Work out the finished part from the listing and answer in its coordinate system (mm). Face numbers are marked on the shaded views. A direction names the side the tool comes from. Coordinates: 2 decimals unless noted, no trailing zeros. Order: outer loops, then holes, each group sorted by start corner. A loop starts at its lowest first (then second) coordinate and runs counter-clockwise, first axis right, second up. Notation, with made-up numbers: (66, -21.75) - (93, -21.75) arc R22 ccw to (93, -2.75) - close; hole circle Ø7 at (75, 43.5). An arc over 180 degrees is marked (long way). Use CSV: the item, a comma, the result in double quotes. Start each with the question number.
from build123d import *

# Parameters (mm, degrees)
SKETCH1_R                 = 1.45
BOSS_EXTRUDE1_DEPTH       = 3
SKETCH4_W                 = 3.5
SKETCH4_H                 = 12
BOSS_EXTRUDE3_DEPTH       = 10.5
SKETCH5_W                 = 2
SKETCH5_H                 = 12
BOSS_EXTRUDE4_DEPTH       = 1.1
SKETCH6_W                 = 0.2
SKETCH6_H                 = 3
BOSS_EXTRUDE5_DEPTH       = 0.5
CHAMFER1_SIZE             = 10.5
F_3_0MM_DOWEL_HOLE1_D     = 2.9
F_3_0MM_DOWEL_HOLE1_DEPTH = 13.5
SKETCH10_R                = 1.45
BOSS_EXTRUDE6_DEPTH       = 3
CUT_EXTRUDE1_START        = -2
SKETCH11_R                = 1.45
CUT_EXTRUDE1_DEPTH        = 2
SKETCH12_R                = 2
CUT_EXTRUDE2_DEPTH        = 8


with BuildPart() as part:
    # Sketch1 → Boss-Extrude1 (new body)
    with BuildSketch(Plane(origin=(0, 0, 0), x_dir=(1, 0, 0), z_dir=(0, 1, 0))):
        with BuildLine():
            Line((-49, 6), (49, 6))
            ThreePointArc((49, 6), (55, 0), (49, -6))
            Line((49, -6), (-49, -6))
            ThreePointArc((-49, -6), (-55, 0), (-49, 6))
        make_face()
        with Locations(Location((-51.5, 0, 0), (0, 0, 270))):
            Circle(SKETCH1_R, mode=Mode.SUBTRACT)
        with Locations(Location((51.5, 0, 0), (0, 0, 270))):
            Circle(SKETCH1_R, mode=Mode.SUBTRACT)
    extrude(amount=BOSS_EXTRUDE1_DEPTH)

    # Sketch4 → Boss-Extrude3 (add)
    with BuildSketch(Plane.XZ):
        with Locations((-21.690023983, 0)):
            Rectangle(SKETCH4_W, SKETCH4_H)
        with Locations((21.690023983, 0)):
            Rectangle(SKETCH4_W, SKETCH4_H)
    extrude(amount=BOSS_EXTRUDE3_DEPTH)

    # Sketch5 → Boss-Extrude4 (add)
    with BuildSketch(Plane.XZ):
        with Locations((5, 0)):
            Rectangle(SKETCH5_W, SKETCH5_H)
        Rectangle(SKETCH5_W, SKETCH5_H)
        with Locations((10, 0)):
            Rectangle(SKETCH5_W, SKETCH5_H)
        with Locations((-5, 0)):
            Rectangle(SKETCH5_W, SKETCH5_H)
        with Locations((-10, 0)):
            Rectangle(SKETCH5_W, SKETCH5_H)
    extrude(amount=BOSS_EXTRUDE4_DEPTH)

    # Sketch6 → Boss-Extrude5 (add)
    with BuildSketch(Plane.XY.offset(6)):
        with Locations((48.9, 1.5)):
            Rectangle(SKETCH6_W, SKETCH6_H)
        with Locations((-48.9, 1.5)):
            Rectangle(SKETCH6_W, SKETCH6_H)
    extrude(amount=BOSS_EXTRUDE5_DEPTH)

    # Chamfer1
    chamfer1_edges = [part.edges().sort_by_distance(p)[0] for p in [
        (-23.440023983, 0, 0),
        (23.440023983, 0, 0),
    ]]
    chamfer(chamfer1_edges, length=CHAMFER1_SIZE - 0.0001)  # a hair under: the kernel refuses the full size

    # Ø3.0mm Dowel Hole1
    with Locations(Plane(origin=(0, 3, 0), x_dir=(1, 0, 0), z_dir=(0, 1, 0))):
        with Locations((-51.5, 0), (51.5, 0)):
            Hole(F_3_0MM_DOWEL_HOLE1_D / 2, depth=F_3_0MM_DOWEL_HOLE1_DEPTH)

    # Sketch10 → Boss-Extrude6 (add)
    # profile 1 of 2: a face of its own
    with BuildSketch(Plane(origin=(0, 3, 0), x_dir=(1, 0, 0), z_dir=(0, 1, 0))):
        with BuildLine():
            Line((-48.8, -6), (-27.05, -6))
            Line((-27.05, -6), (-27.05, 6))
            Line((-27.05, 6), (-49, 6))
            ThreePointArc((-49, 6), (-55, 0), (-49, -6))
            Line((-49, -6), (-49, -6.5))
            Line((-49, -6.5), (-48.8, -6.5))
            Line((-48.8, -6.5), (-48.8, -6))
        make_face()
        with Locations(Location((-51.5, 0, 0), (0, 0, 270.000000001))):
            Circle(SKETCH10_R, mode=Mode.SUBTRACT)
    # profile 2 of 2: a face of its own
    with BuildSketch(Plane(origin=(0, 3, 0), x_dir=(1, 0, 0), z_dir=(0, 1, 0))):
        with BuildLine():
            Line((27.05, 6), (27.05, -6))
            Line((27.05, -6), (48.8, -6))
            Line((48.8, -6), (48.8, -6.5))
            Line((48.8, -6.5), (49, -6.5))
            Line((49, -6.5), (49, -6))
            ThreePointArc((49, -6), (55, 0), (49, 6))
            Line((49, 6), (27.05, 6))
        make_face()
        with Locations(Location((51.5, 0, 0), (0, 0, 270))):
            Circle(SKETCH10_R, mode=Mode.SUBTRACT)
    extrude(amount=BOSS_EXTRUDE6_DEPTH)

    # Sketch11 → Cut-Extrude1 (cut)
    # profile 1 of 2: a face of its own
    with BuildSketch(Plane(origin=(0, 6, 0), x_dir=(1, 0, 0), z_dir=(0, 1, 0)).offset(CUT_EXTRUDE1_START)):
        Polygon((53.491858429, 3.45), (55.483716857, 0), (53.491858429, -3.45), (49.508141571, -3.45), (47.516283143, 0), (49.508141571, 3.45), align=None)
    # profile 2 of 2: a face of its own
    with BuildSketch(Plane(origin=(0, 6, 0), x_dir=(1, 0, 0), z_dir=(0, 1, 0)).offset(CUT_EXTRUDE1_START)):
        Polygon((-47.516283143, 0), (-49.508141571, 3.45), (-53.491858429, 3.45), (-55.483716857, 0), (-53.491858429, -3.45), (-49.508141571, -3.45), align=None)
        with Locations(Location((-51.5, 0, 0), (0, 0, 270.000000001))):
            Circle(SKETCH11_R, mode=Mode.SUBTRACT)
    extrude(amount=CUT_EXTRUDE1_DEPTH, mode=Mode.SUBTRACT)

    # Sketch12 → Cut-Extrude2 (cut)
    with BuildSketch(Plane(origin=(0, 3, 0), x_dir=(1, 0, 0), z_dir=(0, 1, 0))):
        with Locations(Location((-22.5, 0, 0), (0, 0, 270))):
            Circle(SKETCH12_R)
        with Locations(Location((22.5, 0, 0), (0, 0, 270))):
            Circle(SKETCH12_R)
    extrude(amount=-CUT_EXTRUDE2_DEPTH, mode=Mode.SUBTRACT)


solid = part.part
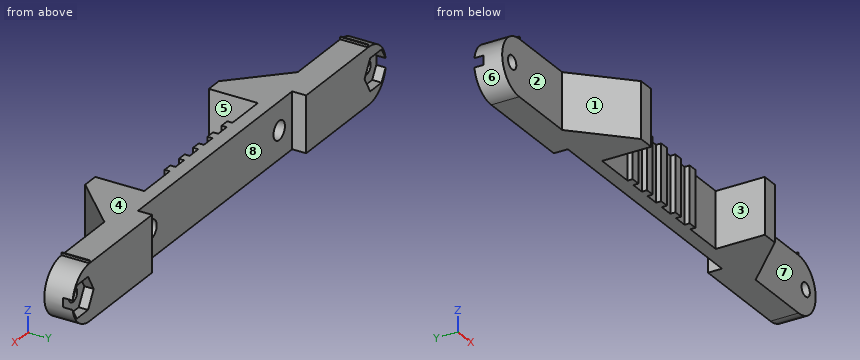
1) The part is cut by section D-D on x = -39. Determine the outline of the cut face in (y, z), plus the area to 3 significant figures.
2) Straight lines are drawn through the part: line 1 (X direction, y = 2, z = 0); line 2 (X direction, y = -2, z = 0); line 3 (X direction, y = 5, z = 3.25). For each, find the intervals that lie inside material, in ascending order. Write a range as [from, to].
3) The part is cut by section B-B on y = -7. Determine the outline of the cut face in (x, z), plus the area to 3 significant figures.
4) The part is cut by section C-C on x = -51.5. Determine the outline of the cut face in (y, z).
5) Flat-ended cylindrical pins translate along their axes: P1, Ø1.5, axis at y = -6, z = 4.5, coming from the +X side; P2, Ø8, axis at x = 44, y = 2, coming from the +Z side; P3, Ø0.6, axis at x = 51, y = 5.5, coming from the -Z side; P4, Ø2.5, axis at x = -51.5, z = 0, coming from the -Y side. Find the tip coordinate at first contact, or state that the pin passes through.
6) For a pull along X with two mould halves and no side action, classify the marked faces 1, 2 and 3 as +X half, -X half, draft (parallel to the pull), parting line (faces both ways), or undercut.
7) The part is cut by section A-A on x = 22.5. Determine the outline of the cut face in (y, z), plus the area to 3 significant figures.
8) For the marked faces 4, 5, 6, 7 and 8, determine the directions among +Z, -Z, +X, -X, +Y, -Y from which every point of the face is accessible in a straight line to the end or side of a thin tool.
Answer key:
1,outline,"(0, -6) - (6, -6) - (6, 6) - (0, 6) - close"
1,area,"72.0 mm^2"
2,line 1,"[-55, -52.95], [-50.05, -24.5], [-20.5, 20.5], [24.5, 50.05], [52.95, 55]"
2,line 2,"[-31.94, -24.5], [-20.5, -19.94], [19.94, 20.5], [24.5, 31.94]"
2,line 3,"[-54.04, -53.61], [-49.39, -27.05], [27.05, 49.39], [53.61, 54.04]"
3,outline,"(-26.94, -6) - (-19.94, -6) - (-19.94, 6) - (-26.94, 6) - close; (19.94, -6) - (26.94, -6) - (26.94, 6) - (19.94, 6) - close"
3,area,"168 mm^2"
4,outline,"(0, -5.45) - (6, -5.45) - (6, -3.45) - (4, -3.45) - (4, -1.45) - (0, -1.45) - close; (0, 1.45) - (4, 1.45) - (4, 3.45) - (6, 3.45) - (6, 5.45) - (0, 5.45) - close"
5,P1,"x = 28.69"
5,P2,"z = 6"
5,P3,"z = -5.75"
5,P4,"through"
6,face 1,"-X half"
6,face 2,"draft"
6,face 3,"undercut"
7,outline,"(-10.5, -6) - (3, -6) - (3, -2) - (-5, -2) - (-5, 2) - (3, 2) - (3, 6) - (-10.5, 6) - close"
7,area,"130 mm^2"
8,face 4,"+Z, +Y, -Y"
8,face 5,"+Z, -Z, -Y"
8,face 6,"-X, +Y, -Y"
8,face 7,"+Z, -Z, +X, -Y"
8,face 8,"+Z, -Z, +Y"
